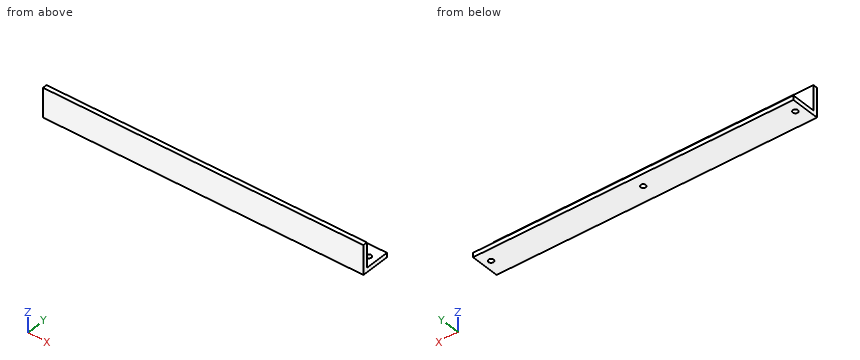
```python
from build123d import *

# Parameters (mm, degrees)
F1_DEPTH = 220
F2_R     = 1.75
F3_DEPTH = 25


with BuildPart() as f1:
    # F0 (on Right) → F1 (new body)
    with BuildSketch(Plane.YZ):
        Polygon((0, 20), (0, 0), (20, 0), (20, 3), (3, 3), (3, 20), align=None)
    extrude(amount=F1_DEPTH)

    # F2 (on face) → F3 (cut)
    with BuildSketch(Plane(origin=(0, 0, 0), x_dir=(1, 0, 0), z_dir=(0, 0, -1))):
        with Locations((5.5, -11.5)):
            Circle(F2_R)
        with Locations((110, -11.5)):
            Circle(F2_R)
        with Locations((214.5, -11.5)):
            Circle(F2_R)
    extrude(amount=-F3_DEPTH, mode=Mode.SUBTRACT)


solid = f1.part
```
The listing builds one solid part. Answer for the finished solid, in the listing's coordinates (mm). Coordinates: 2 decimals unless noted, no trailing zeros. Write each loop counter-clockwise with the first axis right and the second up, starting at its lowest first coordinate (ties: lowest second). Pieces come first, ordered by that corner, then holes. Notation, with made-up numbers: M 8.5,56 L 39.5,56 A17 ccw 39.5,84 Z; hole C -25.75,89 d11. An arc over 180 degrees is marked long. Use a Markdown table: item, result. Add a question column.
1. Given P1, Ø12, axis at x = 60.5, y = 14, coming from the +Z side; P2, Ø5, axis at x = 145.5, z = 10, coming from the +Y side, each flat-ended and moving along its own axis, determine where each tip first touches the part or whether it passes through.
2. Straight lines are drawn through the part: line 1 along X through (y, z) = (11.5, 2); line 2 along Y through (x, z) = (110, 0.6); line 3 along Y through (x, z) = (87.5, 3.5). For each, find the intervals that lie inside material, in ascending order. Write a range as [from, to].
3. Section A-A (x = 124.5) is taken. Give the vertices of the cut face in (y, z).
4. Section B-B (y = 17) is taken. Give the vertices of the cut face in (x, z), plus the area to 3 significant figures.
Data:
| question | item | result |
|---|---|---|
| 1 | P1 | stops at z = 3 |
| 1 | P2 | stops at y = 3 |
| 2 | line 1 | x = [0, 3.75], [7.25, 108.25], [111.75, 212.75], [216.25, 220] |
| 2 | line 2 | y = [0, 9.75], [13.25, 20] |
| 2 | line 3 | y = [0, 3] |
| 3 | outline | M 0,0 L 20,0 L 20,3 L 3,3 L 3,20 L 0,20 Z |
| 4 | outline | M 0,0 L 220,0 L 220,3 L 0,3 Z |
| 4 | area | 660 mm2 |
